Source: CAD feature listing. Evaluate the final solid. Frame: model axes, mm. Give positions to 0.01 mm unless a question says otherwise; leave off trailing zeros. Order: outer loops, then holes, each group sorted by start corner. A loop starts at its lowest first (then second) coordinate and runs counter-clockwise, first axis right, second up. Notation, with made-up numbers: (53.5, 76) - (96.5, 76) arc R32 ccw to (96.5, 109) - close; hole circle Ø9 at (36, 12.5). An arc over 180 degrees is marked (long way). Use CSV: the item, a comma, the result in double quotes.
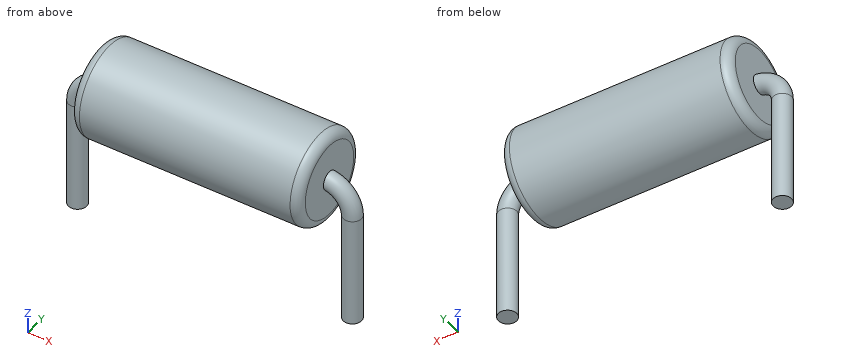
```python
from build123d import *

# Parameters (mm, degrees)
F0_W = 6.35
F0_H = 1.27
F2_R = 0.254
F5_R = 0.254


with BuildPart() as f1:
    # F0 (on Front) → F1 (revolve)
    with BuildSketch(Plane.XZ):
        with Locations((0, 0.635)):
            Rectangle(F0_W, F0_H)
    revolve(axis=Axis((0, 0, 0), (1, 0, 0)))

    # F2
    f2_edges = [f1.edges().sort_by_distance(p)[0] for p in [
        (3.175, 0, -1.27),
        (-3.175, 0, -1.27),
    ]]
    fillet(f2_edges, radius=F2_R)

    # F6: sweep along a path in F3
    with BuildLine(Plane.XZ) as f6_path:
        Line((-3.81, -3.81), (-3.81, -0.762))
        ThreePointArc((-3.81, -0.762), (-3.5868153673, -0.2231846327), (-3.048, 0))
        Line((-3.048, 0), (3.048, 0))
        ThreePointArc((3.048, 0), (3.5868153673, -0.2231846327), (3.81, -0.762))
        Line((3.81, -0.762), (3.81, -3.81))
    # F5 (on offset) → F6 (sweep)
    with BuildSketch(Plane.XY.offset(-3.81)):
        with Locations((-3.81, 0)):
            Circle(F5_R)
    sweep(path=f6_path.line)


solid = f1.part
```
Item 1: Section C-C on y = 0. Return the cut outline in (x, z) (3 decimals).
Filled in:
outline,"(-4.064, -3.81) - (-3.556, -3.81) - (-3.556, -0.762) arc R0.508 cw to (-3.175, -0.27) - (-3.175, -1.016) arc R0.254 ccw to (-2.921, -1.27) - (2.921, -1.27) arc R0.254 ccw to (3.175, -1.016) - (3.175, -0.27) arc R0.508 cw to (3.556, -0.762) - (3.556, -3.81) - (4.064, -3.81) - (4.064, -0.762) arc R1.016 ccw to (3.175, 0.246) - (3.175, 1.016) arc R0.254 ccw to (2.921, 1.27) - (-2.921, 1.27) arc R0.254 ccw to (-3.175, 1.016) - (-3.175, 0.246) arc R1.016 ccw to (-4.064, -0.762) - close"
Item 2: Section A-A on x = 2.75. Return the cut outline in (y, z).
Filled in:
outline,"circle Ø2.54 at (0, 0)"
Item 3: Material intervals for line 1 (X direction, y = 0.05, z = -1.1); line 2 (X direction, y = -0.6, z = -0.05) (3 decimals); line 3 (X direction, y = 0.05, z = -1.3), sorted ascending. Write a range as from..to.
Filled in:
line 1,"x = -4.06..-3.56, -3.16..3.16, 3.56..4.06"
line 2,"x = -3.175..3.175"
line 3,"x = -4.06..-3.56, 3.56..4.06"
Item 4: First-contact query: pin 1 (2 mm diameter, centred on x = -3, z = -2.5, fed in from +Y); pin 2 (1 mm diameter, centred on y = 0.5, z = -0.5, fed in from -X); pin 3 (0.6 mm diameter, centred on y = 0, z = 0, fed in from +X). Flat tips, straight axial feed; report the tip coordinate or a pass-through.
Filled in:
pin 1,"stops at y = 0.25"
pin 2,"stops at x = -4.06"
pin 3,"stops at x = 3.95"
Item 5: Section B-B on z = -1.75. Return the cut outline in (x, y).
Filled in:
outline,"circle Ø0.51 at (-3.81, 0); circle Ø0.51 at (3.81, 0)"
